The model under review builds one solid part; all positions refer to its coordinate system, in mm. A direction names the side the tool comes from. Coordinates: 2 decimals unless noted, no trailing zeros. Loops run counter-clockwise (first coordinate to the right, second up) from the corner with the lowest first, then second, coordinate; pieces in that order, holes last. Notation, with made-up numbers: (56, 81.25) - (112, 81.25) arc R10 cw to (112, 98.25) - close; hole circle Ø8 at (26, 57). An arc over 180 degrees is marked (long way). Use a Markdown table: item, result. Add a question column.
1) To check wall thickness, follow L1, parallel to Z at x = 24, y = 2; L2, parallel to Z at x = 0, y = 31.5. State the ranges of each line that lie inside material, in increasing order. Write a range as [from, to].
2) Add section C-C, the plane z = 0. Give the boundary of the cut face in (x, y), and give its area (3 significant figures).
3) For faces 4 (the flat face through (31.75, 3, 0)), 5 (the cylindrical face through (-23.016, 27.487, -7.248)), list the 3-axis set-ups (+Z, -Z, +X, -X, +Y, -Y) from which the entire face can be reached by the end or side of a thin tool; tool diameter is ignored.
4) The part is to be moulded in two halves that separate along X. For faces 1 (the flat face through (-18, 49.225, 7)), 2 (the flat face through (-31.75, 3, 0)), 3 (the cylindrical face through (27.15, 3.13, 26.45)), say which applies: pulls with the +X half, pulls with the -X half, needs draft (parallel to the pull), parting line crosses it, or undercut.
5) Clearance check with flat-ended pins moving along their axes: pin 1 (3 mm diameter, centred on x = -9, y = 8, fed in from -Z); pin 2 (1.5 mm diameter, centred on x = -21.5, y = 13, fed in from -Z); pin 3 (6 mm diameter, centred on x = -8, y = 36, fed in from -Z); pin 4 (19 mm diameter, centred on x = -2.5, z = 7, fed in from +Y). State where each tip first meets the part, or that it passes through.
6) Add section A-A, the plane x = 0. Give the boundary of the cut face in (y, z), and give its area (3 significant figures).
7) Add section B-B, the plane y = 5.5. Give the boundary of the cut face in (x, z), and give its area (3 significant figures).
8) Add section D-D, the plane z = -27. Give the boundary of the cut face in (x, y).
Autodesk Inventor part; units mm, degrees
ref_plane "YZ Plane" through (0, 0, 0) normal (1, 0, 0) x (0, 1, 0)
ref_plane "XZ Plane" through (0, 0, 0) normal (0, 1, 0) x (-1, 0, 0)
ref_plane "XY Plane" through (0, 0, 0) normal (0, 0, 1) x (1, 0, 0)
sketch "Sketch1" plane through (0, 0, 0) normal (0, 1, 0) x (-1, 0, 0)
  circle A0 centre (0, 0) radius 19.05
  circle A1 centre (0, 0) radius 24.13
  line L0 (31.75, 31.75) -> (-31.75, 31.75)
  line L1 (-31.75, 31.75) -> (-31.75, -31.75)
  line L2 (-31.75, -31.75) -> (31.75, -31.75)
  line L3 (31.75, -31.75) -> (31.75, 31.75)
  line L4 (31.75, 31.75) -> (24.13, 31.75)
  circle A2 centre (24.13, 24.13) radius 3.81
  circle A3 centre (-24.13, 24.13) radius 3.81
  circle A4 centre (24.13, -24.13) radius 3.81
  circle A5 centre (-24.13, -24.13) radius 3.81
  dimension "d10" = 63.5
  dimension "d11" = 63.5
  dimension "d14" = 7.62
extrude "Extrusion1" add sketch "Sketch1" along normal blind 49.2252 contours A1
extrude "Extrusion3" add sketch "Sketch1" along normal blind 6.35 contours A1 | L3 L2 L1 L0 | A2 | A3 | A4 | A5
extrude "Extrusion4" cut sketch "Sketch1" along normal blind 6.35 contours A2 | A3 | A4 | A5
properties part number "Cylinders"
From the geometry:
| question | item | result |
|---|---|---|
| 1 | L1 | z = [-31.75, -27.94], [-20.32, 20.32], [27.94, 31.75] |
| 1 | L2 | z = [-24.13, -19.05], [19.05, 24.13] |
| 2 | outline | (-31.75, 0) - (-19.05, 0) - (-19.05, 49.23) - (-24.13, 49.23) - (-24.13, 6.35) - (-31.75, 6.35) - close; (19.05, 0) - (31.75, 0) - (31.75, 6.35) - (24.13, 6.35) - (24.13, 49.23) - (19.05, 49.23) - close |
| 2 | area | 597 mm^2 |
| 3 | face 4 | +Z, -Z, +X, +Y, -Y |
| 3 | face 5 | +Y |
| 4 | face 1 | needs draft |
| 4 | face 2 | pulls with the -X half |
| 4 | face 3 | undercut |
| 5 | pin 1 | stops at z = -22.93 |
| 5 | pin 2 | stops at z = -12.32 |
| 5 | pin 3 | stops at z = -23.61 |
| 5 | pin 4 | passes through |
| 6 | outline | (0, -31.75) - (6.35, -31.75) - (6.35, -24.13) - (49.23, -24.13) - (49.23, -19.05) - (0, -19.05) - close; (0, 19.05) - (49.23, 19.05) - (49.23, 24.13) - (6.35, 24.13) - (6.35, 31.75) - (0, 31.75) - close |
| 6 | area | 597 mm^2 |
| 7 | outline | (-31.75, -31.75) - (31.75, -31.75) - (31.75, 31.75) - (-31.75, 31.75) - close; hole circle Ø7.62 at (-24.13, -24.13); hole circle Ø7.62 at (-24.13, 24.13); hole circle Ø38.1 at (0, 0); hole circle Ø7.62 at (24.13, -24.13); hole circle Ø7.62 at (24.13, 24.13) |
| 7 | area | 2,710 mm^2 |
| 8 | outline | (-31.75, 0) - (-26.64, 0) - (-26.64, 6.35) - (-31.75, 6.35) - close; (-21.62, 0) - (21.62, 0) - (21.62, 6.35) - (-21.62, 6.35) - close; (26.64, 0) - (31.75, 0) - (31.75, 6.35) - (26.64, 6.35) - close |
